```python
from build123d import *

# Parameters (mm, degrees)
ESQUISSE1_W             = 106
ESQUISSE1_H             = 317
ESQUISSE1_R             = 3.5
BOSS_EXTRU_1_DEPTH      = 2
ESQUISSE3_R             = 1.375
ENL_V_MAT_EXTRU_1_DEPTH = 3
CHANFREIN1_SIZE         = 15
CHANFREIN1_SIZE2        = 25.980762114
ESQUISSE4_R             = 1.25
ESQUISSE4_W             = 56
ESQUISSE4_H             = 26
ENL_V_MAT_EXTRU_2_DEPTH = 10
CONG_1_R                = 10
ESQUISSE5_W             = 40.5
ESQUISSE5_H             = 76
ENL_V_MAT_EXTRU_3_DEPTH = 10
CONG_2_R                = 10
ESQUISSE6_R             = 1.25
ESQUISSE6_W             = 20
ESQUISSE6_H             = 2
ESQUISSE6_W_2           = 2
ESQUISSE6_H_2           = 10
ENL_V_MAT_EXTRU_4_DEPTH = 10
ESQUISSE7_R             = 8
ENL_V_MAT_EXTRU_5_DEPTH = 10
ESQUISSE8_OUTSIDE_W     = 174.852
ESQUISSE8_OUTSIDE_H     = 385.852
ENL_V_MAT_EXTRU_6_DEPTH = 10
ESQUISSE9_R             = 3.5
ENL_V_MAT_EXTRU_7_DEPTH = 10


with BuildPart() as part:
    # Esquisse1 → Boss.-Extru.1 (new body)
    with BuildSketch(Plane(origin=(0, 0, 0), x_dir=(1, 0, 0), z_dir=(0, 1, 0))):
        with Locations((0, 10)):
            Rectangle(ESQUISSE1_W, ESQUISSE1_H)
        with Locations((-33, 128.5)):
            Circle(ESQUISSE1_R, mode=Mode.SUBTRACT)
        with Locations((-33, -128.5)):
            Circle(ESQUISSE1_R, mode=Mode.SUBTRACT)
        with Locations((33, 128.5)):
            Circle(ESQUISSE1_R, mode=Mode.SUBTRACT)
        with Locations((33, -128.5)):
            Circle(ESQUISSE1_R, mode=Mode.SUBTRACT)
    extrude(amount=BOSS_EXTRU_1_DEPTH)

    # Esquisse3 → Enlèv. mat.-Extru.1 (cut, through all)
    with BuildSketch(Plane(origin=(0, 2, 0), x_dir=(1, 0, 0), z_dir=(0, 1, 0))):
        with Locations((-22, -3.5)):
            Circle(ESQUISSE3_R)
        with Locations((-22, 82.5)):
            Circle(ESQUISSE3_R)
        with Locations((36, 82.5)):
            Circle(ESQUISSE3_R)
        with Locations((36, -3.5)):
            Circle(ESQUISSE3_R)
    extrude(amount=-ENL_V_MAT_EXTRU_1_DEPTH, mode=Mode.SUBTRACT)

    # Chanfrein1
    chanfrein1_edges = [part.edges().sort_by_distance(p)[0] for p in [
        (-53, 1, -168.5),
        (53, 1, -168.5),
    ]]
    chanfrein1_side = [part.faces().sort_by_distance(p)[0] for p in [
        (0, 1, -168.5),
    ]]
    chamfer(chanfrein1_edges, length=CHANFREIN1_SIZE, length2=CHANFREIN1_SIZE2, reference=chanfrein1_side[0])

    # Esquisse4 → Enlèv. mat.-Extru.2 (cut)
    with BuildSketch(Plane(origin=(0, 2, 0), x_dir=(1, 0, 0), z_dir=(0, 1, 0))):
        with Locations((38, -63.5)):
            Circle(ESQUISSE4_R)
        with Locations((38, -27.5)):
            Circle(ESQUISSE4_R)
        with Locations((-38, -63.5)):
            Circle(ESQUISSE4_R)
        with Locations((-38, -27.5)):
            Circle(ESQUISSE4_R)
        with Locations((0, -45.5)):
            Rectangle(ESQUISSE4_W, ESQUISSE4_H)
    extrude(amount=-ENL_V_MAT_EXTRU_2_DEPTH, mode=Mode.SUBTRACT)

    # Congé1
    cong_1_edges = [part.edges().sort_by_distance(p)[0] for p in [
        (-28, 1, 58.5),
        (-28, 1, 32.5),
        (28, 1, 32.5),
        (28, 1, 58.5),
    ]]
    fillet(cong_1_edges, radius=CONG_1_R)

    # Esquisse5 → Enlèv. mat.-Extru.3 (cut)
    with BuildSketch(Plane(origin=(0, 2, 0), x_dir=(1, 0, 0), z_dir=(0, 1, 0))):
        with Locations((3.25, 39.5)):
            Rectangle(ESQUISSE5_W, ESQUISSE5_H)
    extrude(amount=-ENL_V_MAT_EXTRU_3_DEPTH, mode=Mode.SUBTRACT)

    # Congé2
    cong_2_edges = [part.edges().sort_by_distance(p)[0] for p in [
        (-17, 1, -1.5),
        (-17, 1, -77.5),
        (23.5, 1, -77.5),
        (23.5, 1, -1.5),
    ]]
    fillet(cong_2_edges, radius=CONG_2_R)

    # Esquisse6 → Enlèv. mat.-Extru.4 (cut)
    with BuildSketch(Plane(origin=(0, 2, 0), x_dir=(1, 0, 0), z_dir=(0, 1, 0))):
        with Locations((-15, 113.5)):
            Circle(ESQUISSE6_R)
        with Locations((15, 113.5)):
            Circle(ESQUISSE6_R)
        with Locations((-15, 143.5)):
            Circle(ESQUISSE6_R)
        with Locations((15, 143.5)):
            Circle(ESQUISSE6_R)
        with Locations((0, 128.5)):
            Rectangle(ESQUISSE6_W, ESQUISSE6_H)
        with Locations((-0.179881847, 119.5)):
            Rectangle(ESQUISSE6_W_2, ESQUISSE6_H_2)
    extrude(amount=-ENL_V_MAT_EXTRU_4_DEPTH, mode=Mode.SUBTRACT)

    # Esquisse7 → Enlèv. mat.-Extru.5 (cut)
    with BuildSketch(Plane(origin=(0, 2, 0), x_dir=(1, 0, 0), z_dir=(0, 1, 0))):
        with Locations((0, -91.5)):
            Circle(ESQUISSE7_R)
        with Locations((-26.5, -91.5)):
            Circle(ESQUISSE7_R)
        with Locations((26.5, -91.5)):
            Circle(ESQUISSE7_R)
    extrude(amount=-ENL_V_MAT_EXTRU_5_DEPTH, mode=Mode.SUBTRACT)

    # Esquisse8 outside → Enlèv. mat.-Extru.6 (cut)
    with BuildSketch(Plane(origin=(0, 2, 0), x_dir=(1, 0, 0), z_dir=(0, 1, 0))):
        with Locations((0, 10)):
            Rectangle(ESQUISSE8_OUTSIDE_W, ESQUISSE8_OUTSIDE_H)
        with BuildLine():
            Line((38, 168.5), (-38, 168.5))
            Line((-38, 168.5), (-53, 142.519237886))
            Line((-53, 142.519237886), (-53, -91.5))
            Line((-53, -91.5), (-42.675385347, -131.027235323))
            ThreePointArc((-42.675385347, -131.027235323), (-39.11259547, -136.41430203), (-33, -138.5))
            Line((-33, -138.5), (33, -138.5))
            ThreePointArc((33, -138.5), (39.11259547, -136.41430203), (42.675385347, -131.027235323))
            Line((42.675385347, -131.027235323), (53, -91.5))
            Line((53, -91.5), (53, 142.519237886))
            Line((53, 142.519237886), (38, 168.5))
        make_face(mode=Mode.SUBTRACT)
    extrude(amount=-ENL_V_MAT_EXTRU_6_DEPTH, mode=Mode.SUBTRACT)

    # Esquisse9 → Enlèv. mat.-Extru.7 (cut)
    with BuildSketch(Plane(origin=(0, 2, 0), x_dir=(1, 0, 0), z_dir=(0, 1, 0))):
        with Locations((45, 10.423949842)):
            Circle(ESQUISSE9_R)
        with Locations((-45, 10.423949842)):
            Circle(ESQUISSE9_R)
    extrude(amount=-ENL_V_MAT_EXTRU_7_DEPTH, mode=Mode.SUBTRACT)


solid = part.part
```
Geometry: final body of the model. Coordinates: model frame, mm. A direction names the side the tool comes from. Round coordinates to 2 decimals unless told otherwise and drop trailing zeros. Loops run counter-clockwise (first coordinate to the right, second up) from the corner with the lowest first, then second, coordinate; pieces in that order, holes last.
Item 1: Line query: L1, parallel to Z at x = 12, y = 0.25; L2, parallel to Z at x = -1, y = 1.5; L3, parallel to Z at x = 35, y = 0.95. Output: solid intervals per line, ascending.
Checked values:
L1: z = -168.5 to -77.5, -1.5 to 32.5, 58.5 to 138.5
L2: z = -168.5 to -129.5, -127.5 to -124.5, -114.5 to -77.5, -1.5 to 32.5, 58.5 to 83.56, 99.44 to 138.5
L3: z = -168.5 to -131.37, -125.63 to -83.44, -81.56 to 2.56, 4.44 to 125.63, 131.37 to 138.3
Item 2: Section A-A, the plane z = -43.5. Output: boundary loops of the cut face in (x, y).
Checked values:
outline: (-53, 0) - (-17, 0) - (-17, 2) - (-53, 2) - close; (23.5, 0) - (53, 0) - (53, 2) - (23.5, 2) - close
Item 3: Section B-B, the plane y = 1.25. State how many separate pieces and enclosed holes the cut face has, plus the area to 3 significant figures.
Checked values:
separate pieces: 1
enclosed holes: 25
area: 26,200 mm2
Item 4: Mould query, pull axis Z, two halves, no side actions, for faces 1 (the cylindrical face through (24.99, 0.99, 55.65)), 2 (the cylindrical face through (-39.185, 1.014, 136.358)), 3 (the flat face through (45.605, 0.986, -155.328)). Classes: released by +Z, released by -Z, zero draft, split by the parting line, or undercut.
Checked values:
face 1: undercut
face 2: released by +Z
face 3: released by -Z
Item 5: Reachability of faces 4 (the flat face through (-45.605, 0.986, -155.328)), 5 (the cylindrical face through (20.49, 0.99, -4.35)) from +Z, -Z, +X, -X, +Y, -Y: full face, straight path, thin tool, end or side. Return the list, or none.
Checked values:
face 4: -Z, -X, +Y, -Y
face 5: +Y, -Y
Item 6: Contact query for flat-ended pins moving along their axis: P1, Ø6.5, axis at x = 33, z = 128.5, coming from the -Y side; P2, Ø1, axis at x = 34, y = 1, coming from the +Z side. Output: stop coordinate, or through.
Checked values:
P1: passes through
P2: stops at z = 138.49
